from build123d import *

# Parameters (mm, degrees)
SKETCH1_W           = 100
SKETCH1_H           = 50
BOSS_EXTRUDE1_DEPTH = 3
SKETCH2_R           = 6.75
SKETCH2_R_2         = 2.25
CUT_EXTRUDE1_DEPTH  = 56.982140009
FILLET1_R           = 25


with BuildPart() as part:
    # Sketch1 → Boss-Extrude1 (new body)
    with BuildSketch(Plane.XY):
        Rectangle(SKETCH1_W, SKETCH1_H)
    extrude(amount=BOSS_EXTRUDE1_DEPTH)

    # Sketch2 → Cut-Extrude1 (cut, through all)
    with BuildSketch(Plane.XY.offset(3)):
        with Locations((34.310453011, 0)):
            Circle(SKETCH2_R)
        with Locations((-14.393398282, 10.606601718)):
            Circle(SKETCH2_R_2)
        with Locations((-35.606601718, -10.606601718)):
            Circle(SKETCH2_R_2)
    extrude(amount=-CUT_EXTRUDE1_DEPTH, mode=Mode.SUBTRACT)

    # Fillet1
    fillet1_edges = [part.edges().sort_by_distance(p)[0] for p in [
        (-50, -25, 1.5),
        (-50, 25, 1.5),
        (50, 25, 1.5),
        (50, -25, 1.5),
    ]]
    fillet(fillet1_edges, radius=FILLET1_R - 0.0001)  # a hair under: the kernel refuses the full size


solid = part.part
Model file for the job. Use its own axes, mm. Round coordinates to 2 decimals unless told otherwise and drop trailing zeros. Loops run counter-clockwise (first coordinate to the right, second up) from the corner with the lowest first, then second, coordinate; pieces in that order, holes last. Notation, with made-up numbers: M -20,59.5 L 6,59.5 A21 cw 6,70.5 Z; hole C 9.25,-2.75 d1. An arc over 180 degrees is marked long. One line per question, with ' | ' between items.
1) Flat gauge pins, fed straight in: pin 1 (1 mm diameter, centred on x = 29.5, z = 1.5, fed in from -Y); pin 2 (1 mm diameter, centred on y = 10.5, z = 2, fed in from -X); pin 3 (1 mm diameter, centred on y = 3, z = 1, fed in from -X). Where does each tip first touch, or does it go through?
Solved:
pin 1: stops at y = -24.68 | pin 2: stops at x = -47.91 | pin 3: stops at x = -49.87
2) Mould opens along Y. For faces 1 (the flat face through (0, -25, 1)), 2 (the cylindrical face through (-42.871, 17.482, 1.521)), 3 (the cylindrical face through (32.85, -6.59, 1.52)) say: +Y half, -Y half, draft (parallel to the pull), parting line (faces both ways), or undercut.
Solved:
face 1: -Y half | face 2: +Y half | face 3: undercut
3) Band-saw the part on C-C (y = 21). Give the cut face in (x, z).
Solved:
outline: M -38.56,0 L 38.56,0 L 38.56,3 L -38.56,3 Z
4) Drill centre lines: line 1 along Y through (x, z) = (29.5, 1.75); line 2 along X through (y, z) = (6, 1.7); line 3 along X through (y, z) = (-12.5, 1.2). Where is each one in solid material? Low to high.
Solved:
line 1: y = -24.59 to -4.74, 4.74 to 24.59 | line 2: x = -49.27 to 31.22, 37.4 to 49.27 | line 3: x = -46.65 to -36.82, -34.39 to 46.65
5) Band-saw the part on B-B (y = 14). Give the cut face in (x, z), then the cut area to 3 significant figures.
Solved:
outline: M -45.71,0 L 45.71,0 L 45.71,3 L -45.71,3 Z | area: 274 mm²
6) Band-saw the part on A-A (z = 1.3). Give the number of separate pieces and of enclosed holes in the cut face, then the cut area to 3 significant figures.
Solved:
separate pieces: 1 | enclosed holes: 3 | area: 4,290 mm²
